Input: part model. Units: mm. Frame: model coordinates. Face numbers are marked on the shaded views. A direction names the side the tool comes from. Give positions to 0.01 mm unless a question says otherwise; leave off trailing zeros. Loops run counter-clockwise (first coordinate to the right, second up) from the corner with the lowest first, then second, coordinate; pieces in that order, holes last. Notation, with made-up numbers: (-15.5, 1.5) -> (-3.5, 1.5) arc R22 cw to (-3.5, 11.5) -> close; hole circle Ø1 at (33.5, 80.5). An arc over 180 degrees is marked (long way). Use CSV: the item, a comma, the result in double quotes.
```python
from build123d import *

# Parameters (mm, degrees)
SKETCH1_W            = 11.90625
SKETCH1_H            = 1.5
BOSS_EXTRUDE1_DEPTH  = 17.4625
SKETCH3_W            = 9
SKETCH3_H            = 1
SKETCH6_R            = 9.525
BOSS_EXTRUDE2_DEPTH  = 1
M8_CLEARANCE_HOLE1_D = 9.525


with BuildPart() as part:
    # Sketch1 → Revolve1 (revolve)
    with BuildSketch(Plane(origin=(0, 0, 0), x_dir=(-1, 0, 0), z_dir=(0, 0, -1)), mode=Mode.PRIVATE) as revolve1_sk:
        with Locations((-5.953125, -0.75)):
            Rectangle(SKETCH1_W, SKETCH1_H)
    revolve(revolve1_sk.sketch.rotate(Axis((0, -1.5, 0), (0, 1, 0)), 270), axis=Axis((0, -1.5, 0), (0, 1, 0)))

    # Sketch2 → Boss-Extrude1 (add)
    with BuildSketch(Plane(origin=(0, 0, 0), x_dir=(-1, 0, 0), z_dir=(0, 1, 0))):
        Polygon((10.998522628, 0), (5.499261314, -9.525), (-5.499261314, -9.525), (-10.998522628, 0), (-5.499261314, 9.525), (5.499261314, 9.525), align=None)
    extrude(amount=BOSS_EXTRUDE1_DEPTH)

    # Sketch3 → Revolve2 (revolve)
    with BuildSketch(Plane.XY, mode=Mode.PRIVATE) as revolve2_sk:
        with Locations((4.5, 17.9625)):
            Rectangle(SKETCH3_W, SKETCH3_H)
    revolve(revolve2_sk.sketch.rotate(Axis((0, 18.4625, 0), (0, -1, 0)), 270), axis=Axis((0, 18.4625, 0), (0, -1, 0)))

    # Sketch6 → Boss-Extrude2 (add)
    with BuildSketch(Plane(origin=(0, 18.4625, 0), x_dir=(1, 0, 0), z_dir=(0, 1, 0))):
        with Locations(Location((0, 0, 0), (0, 0, 270))):
            Circle(SKETCH6_R)
    extrude(amount=BOSS_EXTRUDE2_DEPTH)

    # M8 Clearance Hole1 (through all)
    with Locations(Plane(origin=(0, -1.5, 0), x_dir=(-1, 0, 0), z_dir=(0, -1, 0))):
        with Locations((0, 0)):
            Hole(M8_CLEARANCE_HOLE1_D / 2)


solid = part.part
```
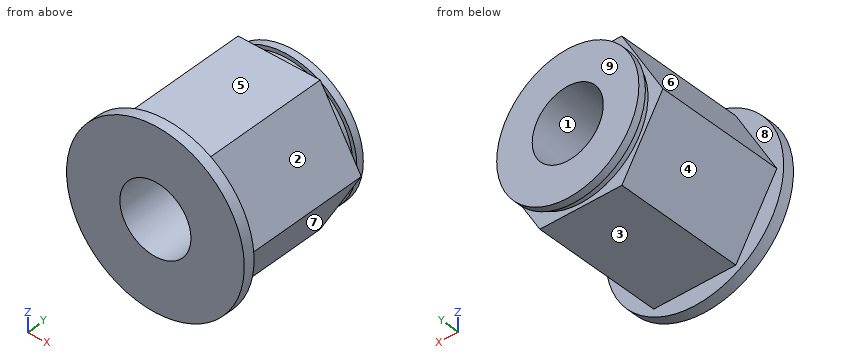
1) Section query B-B (y = 5.5). Return loops of the section in (x, z) (1 decimal), then the cut area to 3 significant figures.
From the geometry:
outline,"(-11, 0) -> (-5.5, -9.5) -> (5.5, -9.5) -> (11, 0) -> (5.5, 9.5) -> (-5.5, 9.5) -> close; hole circle Ø9.5 at (0, 0)"
area,"243 mm^2"
2) Contact query for flat-ended pins moving along their axis: pin 1 (8 mm diameter, centred on y = 16.5, z = -4.5, fed in from +X); pin 2 (3.5 mm diameter, centred on x = 1, y = 4.5, fed in from +Z) (3 decimals); pin 3 (1.5 mm diameter, centred on y = 4.5, z = 9, fed in from -X); pin 4 (5.5 mm diameter, centred on x = 0, z = 0, fed in from -Y). Output: stop coordinate, or through.
From the geometry:
pin 1,"stops at x = 10.71"
pin 2,"stops at z = 9.525"
pin 3,"stops at x = -6.24"
pin 4,"passes through"
3) Section query C-C (z = 8.25). Return loops of the section in (x, y).
From the geometry:
outline,"(-8.58, -1.5) -> (8.58, -1.5) -> (8.58, 0) -> (6.24, 0) -> (6.24, 17.46) -> (3.6, 17.46) -> (3.6, 18.46) -> (4.76, 18.46) -> (4.76, 19.46) -> (-4.76, 19.46) -> (-4.76, 18.46) -> (-3.6, 18.46) -> (-3.6, 17.46) -> (-6.24, 17.46) -> (-6.24, 0) -> (-8.58, 0) -> close"
4) Section query D-D (x = -10). Return loops of the section in (y, z), then the cut area to 3 significant figures.
From the geometry:
outline,"(-1.5, -6.46) -> (0, -6.46) -> (0, -1.73) -> (17.46, -1.73) -> (17.46, 1.73) -> (0, 1.73) -> (0, 6.46) -> (-1.5, 6.46) -> close"
area,"79.8 mm^2"
5) Ray query, line 1 (Z direction, x = 0, y = 10.75) (1 decimal); line 2 (X direction, y = 16.25, z = -3.5); line 3 (X direction, y = 17.75, z = -2.75). Return the intervals inside material, ascending.
From the geometry:
line 1,"z = -9.5 to -4.8, 4.8 to 9.5"
line 2,"x = -8.98 to -3.23, 3.23 to 8.98"
line 3,"x = -8.57 to -3.89, 3.89 to 8.57"
6) Section query A-A (x = 0). Return loops of the section in (y, z) (1 decimal), then the cut area to 3 significant figures.
From the geometry:
outline,"(-1.5, -11.9) -> (0, -11.9) -> (0, -9.5) -> (17.5, -9.5) -> (17.5, -9) -> (18.5, -9) -> (18.5, -9.5) -> (19.5, -9.5) -> (19.5, -4.8) -> (-1.5, -4.8) -> close; (-1.5, 4.8) -> (19.5, 4.8) -> (19.5, 9.5) -> (18.5, 9.5) -> (18.5, 9) -> (17.5, 9) -> (17.5, 9.5) -> (0, 9.5) -> (0, 11.9) -> (-1.5, 11.9) -> close"
area,"206 mm^2"
7) Mould query, pull axis X, two halves, no side actions, for the marked faces 1, 2, 3 and 4. Classes: pulls with the +X half, pulls with the -X half, needs draft (parallel to the pull), parting line crosses it, or undercut.
From the geometry:
face 1,"undercut"
face 2,"pulls with the +X half"
face 3,"needs draft"
face 4,"pulls with the -X half"
8) Reachability of the marked faces 5, 6, 7, 8 and 9 from +Z, -Z, +X, -X, +Y, -Y: full face, straight path, thin tool, end or side. Return the list, or none.
From the geometry:
face 5,"+Z, +X, -X, +Y"
face 6,"+Z, -X, +Y"
face 7,"-Z, +X, +Y"
face 8,"+Y"
face 9,"+Z, -Z, +X, -X, +Y"
